```python
from build123d import *

# Parameters (mm, degrees)
SKETCH4_W               = 45
SKETCH4_H               = 65
BOSS_EXTRUDE2_DEPTH     = 55
CUT_EXTRUDE1_DEPTH      = 52.5
F_1_4_28_TAPPED_HOLE1_D = 5.4102


with BuildPart() as part:
    # Sketch4 → Boss-Extrude2 (new body)
    with BuildSketch(Plane.XY):
        with Locations((-7.784904398, -11.939291809)):
            Rectangle(SKETCH4_W, SKETCH4_H)
    extrude(amount=BOSS_EXTRUDE2_DEPTH)

    # Sketch5 → Cut-Extrude1 (cut)
    with BuildSketch(Plane.XY.offset(55)):
        with BuildLine():
            Line((-28.034904398, -22.189291809), (-28.034904398, -1.689291809))
            ThreePointArc((-28.034904398, -1.689291809), (-7.784904398, 18.560708191), (12.465095602, -1.689291809))
            Line((12.465095602, -1.689291809), (12.465095602, -22.189291809))
            ThreePointArc((12.465095602, -22.189291809), (-7.784904398, -42.439291809), (-28.034904398, -22.189291809))
        make_face()
    extrude(amount=-CUT_EXTRUDE1_DEPTH, mode=Mode.SUBTRACT)

    # 1/4-28 Tapped Hole1 (through all)
    with Locations(Plane(origin=(0, 0, 0), x_dir=(-1, 0, 0), z_dir=(0, 0, -1))):
        with Locations((7.784904398, -16.439291809)):
            Hole(F_1_4_28_TAPPED_HOLE1_D / 2)


solid = part.part
```
Can you work these out from the model? Positions are in its coordinate system, mm. A direction names the side the tool comes from. Round coordinates to 2 decimals unless told otherwise and drop trailing zeros. Loops run counter-clockwise (first coordinate to the right, second up) from the corner with the lowest first, then second, coordinate; pieces in that order, holes last. Notation, with made-up numbers: M 89.5,64.25 L 144.5,64.25 A19 cw 144.5,97.25 Z; hole C 18.25,67 d10. An arc over 180 degrees is marked long. Answer as a JSON object with one key per item and string values. Group by question number.
Q1. Please list where these lines run through material, in increasing order: L1, parallel to X at y = -15, z = 25.5; L2, parallel to Y at x = -7.5, z = 31; L3, parallel to Z at x = 2, y = -9.
Q2. We'd pull the mould along Y, two halves only. Please class faces 3 (the flat face through (-30.285, -12, 27)), 4 (the flat face through (-28.035, -12, 29)), 5 (the flat face through (-8, 20.561, 27)): +Y half, -Y half, draft (parallel to the pull), parting line (faces both ways), or undercut.
Q3. Imagine slicing it at C-C, the plane y = -20. Please give me the cut outline in (x, z), then the cut area to 3 significant figures.
Q4. Imagine slicing it at D-D, the plane x = -16. Please give me the cut outline in (y, z).
Q5. Imagine slicing it at B-B, the plane x = -8. Please give me the cut outline in (y, z), then the cut area to 3 significant figures.
Q6. On a 3-axis mill with a long thin cutter (end or side, diameter ignored), from which of +Z, -Z, +X, -X, +Y, -Y can I reach the whole of each face in a straight line? I mean faces 1 (the flat face through (-8, -44.439, 27)), 2 (the cylindrical face through (-8.23, 18.556, 29.118)). Say none if no direction works.
Q7. Imagine slicing it at A-A, the plane z = 36. Please give me the cut outline in (x, y), then the cut area to 4 significant figures.
Q8. Will this pin go through, and if not, where does the flat tip stop? pin 1 (12 mm diameter, centred on x = -10, y = -1.5, fed in from +Z).
Findings:
{
 "1": {"L1": "x = -30.28 to -28.03, 12.47 to 14.72", "L2": "y = -44.44 to -42.44, 18.56 to 20.56", "L3": "z = 0 to 2.5"},
 "2": {"face 3": "draft", "face 4": "undercut", "face 5": "+Y half"},
 "3": {"outline": "M -30.28,0 L 14.72,0 L 14.72,55 L 12.47,55 L 12.47,2.5 L -28.03,2.5 L -28.03,55 L -30.28,55 Z", "area": "349 mm2"},
 "4": {"outline": "M -44.44,0 L 20.56,0 L 20.56,55 L 16.82,55 L 16.82,2.5 L -40.7,2.5 L -40.7,55 L -44.44,55 Z"},
 "5": {"outline": "M -44.44,0 L -19.14,0 L -19.14,2.5 L -42.44,2.5 L -42.44,55 L -44.44,55 Z; M -13.74,0 L 20.56,0 L 20.56,55 L 18.56,55 L 18.56,2.5 L -13.74,2.5 Z", "area": "359 mm2"},
 "6": {"face 1": "+Z, -Z, +X, -X, -Y", "face 2": "+Z"},
 "7": {"outline": "M -30.28,-44.44 L 14.72,-44.44 L 14.72,20.56 L -30.28,20.56 Z; hole M -28.03,-22.19 A20.25 ccw 12.47,-22.19 L 12.47,-1.69 A20.25 ccw -28.03,-1.69 Z", "area": "806.5 mm2"},
 "8": {"pin 1": "stops at z = 2.5"}
}
